Autodesk Inventor part; units mm, degrees
ref_plane "YZ Plane" through (0, 0, 0) normal (1, 0, 0) x (0, 1, 0)
ref_plane "XZ Plane" through (0, 0, 0) normal (0, 1, 0) x (-1, 0, 0)
ref_plane "XY Plane" through (0, 0, 0) normal (0, 0, 1) x (1, 0, 0)
sketch "Sketch1" plane through (0, 0, 0) normal (0, 0, 1) x (1, 0, 0)
  line L0 (127, 0) -> (127, 50.8)
  line L1 (127, 50.8) -> (0, 50.8)
  line L2 (0, 50.8) -> (0, 0)
  arc A0 (109.5375, 0) -> (68.2625, 0) centre (88.9, 0) ccw
  arc A1 (36.3964, 0) -> (14.4, 0) centre (25.3982, 0) ccw
  line L3 (14.4, 0) -> (0, 0)
  line L4 (127, 0) -> (109.5375, 0)
  line L5 (68.2625, 0) -> (36.3964, 0)
  dimension "d0" = 127
  dimension "d2" = 41.275
  dimension "d25" = 38.1
  dimension "d26" = 21.9964
  dimension "d31" = 31.8661
  dimension "d32" = 14.4
  dimension "d33" = 50.8
extrude "Extrusion1" add sketch "Sketch1" along normal blind 187.96
sketch "Sketch3" plane through (127, 0, 0) normal (1, 0, 0) x (0, 0, -1)
  line L0 (0, 50.8) -> (-187.96, 50.8)
  line L1 (0, 0) -> (-187.96, 0)
  line L2 (-35.56, 38.1) -> (-35.56, 0)
  line L3 (0, 0) -> (-187.96, 0)
  line L4 (-93.98, 0) -> (-93.98, 38.1)
  line L5 (-152.4, 38.1) -> (-152.4, 0)
  line L6 (0, 0) -> (0, 50.8)
  line L7 (-187.96, 0) -> (-175.26, 0)
  line L8 (-175.26, 0) -> (-175.26, 38.1)
  line L9 (-175.26, 50.8) -> (-187.96, 50.8)
  line L10 (-187.96, 50.8) -> (-187.96, 0)
  line L11 (-116.84, 0) -> (-129.54, 0)
  line L12 (-129.54, 0) -> (-129.54, 38.1)
  line L13 (-129.54, 50.8) -> (-116.84, 50.8)
  line L14 (-116.84, 38.1) -> (-116.84, 0)
  line L15 (-35.56, 38.1) -> (-35.56, 0)
  line L16 (0, 0) -> (-12.7, 0)
  line L17 (-12.7, 0) -> (-12.7, 38.1)
  line L18 (-12.7, 50.8) -> (0, 50.8)
  line L19 (0, 50.8) -> (0, 0)
  line L20 (-71.12, 0) -> (-58.42, 0)
  line L21 (-58.42, 0) -> (-58.42, 38.1)
  line L22 (-58.42, 50.8) -> (-71.12, 50.8)
  line L23 (-71.12, 38.1) -> (-71.12, 0)
  line L24 (-187.96, 50.8) -> (-187.96, 0)
  line L25 (-187.96, 50.8) -> (0, 50.8)
  line L26 (-58.42, 38.1) -> (-12.7, 38.1)
  line L27 (-175.26, 38.1) -> (-129.54, 38.1)
  line L28 (-116.84, 38.1) -> (-71.12, 38.1)
  dimension "d15" = 35.56
  dimension "d16" = 93.98
  dimension "d17" = 152.4
  dimension "d18" = 12.7
  dimension "d34" = 38.1
extrude "Extrusion2" cut sketch "Sketch3" against normal blind 187.96 contours L1 L2 L26 L17 | L1 L21 L26 L2 | L1 L4 L28 L23 | L1 L14 L28 L4 | L1 L5 L27 L12 | L8 L27 L5 L1
properties part number "E.Engine Block Bottom"
Can you work these out from the model? Positions are in its coordinate system, mm. A direction names the side the tool comes from. Give positions to 0.01 mm unless a question says otherwise; leave off trailing zeros. Loops run counter-clockwise (first coordinate to the right, second up) from the corner with the lowest first, then second, coordinate; pieces in that order, holes last. Notation, with made-up numbers: M 82.5,51 L 128.5,51 A19 cw 128.5,87 Z; hole C 17.25,62.5 d3. An arc over 180 degrees is marked long. One line per item, written item: value.
1) Imagine slicing it at A-A on z = 69. Write out the boundary of the cut face in (x, y) (1 decimal).
Geometry check:
outline: M 0,0 L 14.4,0 A11 cw 36.4,0 L 68.3,0 A20.6 cw 109.5,0 L 127,0 L 127,50.8 L 0,50.8 Z
2) On a 3-axis mill with a long thin cutter (end or side, diameter ignored), from which of +Z, -Z, +X, -X, +Y, -Y can I reach the whole of each face in a straight line? I mean faces 5 (the face through (63, 31, 0)), 6 (the face through (64, 23, 12.7)). Say none if no direction works.
Geometry check:
face 5: -Z, +X, -X, +Y, -Y
face 6: +X, -X, -Y
3) I'm going to push a flat-ended pin straight in: pin 1 (13.5 mm diameter, centred on x = 59.5, z = 85, fed in from -Y). Where does the tip first touch, or does it pass through?
Geometry check:
pin 1: stops at y = 38.1
4) Please list where these lines run through material, in increasing order: line 1 (Z direction, x = 36, y = 37); line 2 (Y direction, x = 86.5, z = 157.5); line 3 (X direction, y = 14.5, z = 70).
Geometry check:
line 1: z = 0 to 12.7, 58.42 to 71.12, 116.84 to 129.54, 175.26 to 187.96
line 2: y = 38.1 to 50.8
line 3: x = 0 to 74.21, 103.59 to 127
5) Imagine slicing it at D-D on x = 19. Write out the boundary of the cut face in (y, z), and give its area (3 significant figures).
Geometry check:
outline: M 8.95,0 L 50.8,0 L 50.8,187.96 L 8.95,187.96 L 8.95,175.26 L 38.1,175.26 L 38.1,129.54 L 8.95,129.54 L 8.95,116.84 L 38.1,116.84 L 38.1,71.12 L 8.95,71.12 L 8.95,58.42 L 38.1,58.42 L 38.1,12.7 L 8.95,12.7 Z
area: 3,870 mm²
6) Thinking about a two-plate mould opening in X: for faces 1 (the face through (88.446, 20.633, 6.261)), 2 (the face through (25.156, 10.996, 6.261)), 3 (the face through (0, 43, 93)), 4 (the face through (118, 0, 123)), which applies, +X half, -X half, draft (parallel to the pull), parting line (faces both ways), or undercut?
Geometry check:
face 1: undercut
face 2: undercut
face 3: -X half
face 4: draft
7) Imagine slicing it at B-B on x = 88.9. Write out the boundary of the cut face in (y, z).
Geometry check:
outline: M 20.64,0 L 50.8,0 L 50.8,187.96 L 20.64,187.96 L 20.64,175.26 L 38.1,175.26 L 38.1,129.54 L 20.64,129.54 L 20.64,116.84 L 38.1,116.84 L 38.1,71.12 L 20.64,71.12 L 20.64,58.42 L 38.1,58.42 L 38.1,12.7 L 20.64,12.7 Z
8) Imagine slicing it at C-C on y = 8.5. Count the separate pieces of the cut face and the enclosed holes in it, and give its area (3 significant figures).
Geometry check:
separate pieces: 12
enclosed holes: 0
area: 3,830 mm²
